Autodesk Inventor part; units mm, degrees
ref_plane "YZ Plane" through (0, 0, 0) normal (1, 0, 0) x (0, 1, 0)
ref_plane "XZ Plane" through (0, 0, 0) normal (0, 1, 0) x (-1, 0, 0)
ref_plane "XY Plane" through (0, 0, 0) normal (0, 0, 1) x (1, 0, 0)
sketch "Skizze1" plane through (0, 0, 0) normal (0, 0, 1) x (1, 0, 0)
  line L0 (27.5, 0) -> (-27.5, 0)
  line L1 (-27.5, 0) -> (-27.5, 210)
  line L2 (-27.5, 210) -> (27.5, 210)
  line L3 (27.5, 210) -> (27.5, 0)
  line L4 (0, 252) -> (0, -42)
  line L5 (-38.5, 0) -> (38.5, 0)
  point P0 (0, 0)
  point P1 (0, 0)
  dimension "d0" = 210
  dimension "d1" = 55
extrude "Extrusion1" add sketch "Skizze1" along normal blind 10
sketch "Skizze2" plane through (0, 0, 10) normal (0, 0, 1) x (1, 0, 0)
  line L0 (27.5, 210) -> (27.5, 0)
  circle A0 centre (3.5, 195.1) radius 4.3
  circle A1 centre (-6.5, 192.1) radius 1.2295
  circle A2 centre (-6.5, 198.1) radius 1.2295
  line L1 (21.5, 200.1) -> (-17.5, 200.1)
  line L2 (-17.5, 190.1) -> (-17.5, 200.1)
  line L3 (21.5, 190.1) -> (-17.5, 190.1)
  line L4 (21.5, 190.1) -> (21.5, 200.1)
  line L5 (19.1583, 143.6) -> (26.6417, 143.6)
  arc A3 (19.1583, 156.6) -> (19.1583, 143.6) centre (22.9, 150.1) ccw
  line L6 (26.6417, 156.6) -> (19.1583, 156.6)
  arc A4 (26.6417, 143.6) -> (26.6417, 156.6) centre (22.9, 150.1) ccw
  circle A5 centre (3.5, 105.1) radius 4.3
  circle A6 centre (-6.5, 102.1) radius 1.2295
  circle A7 centre (-6.5, 108.1) radius 1.2295
  line L7 (21.5, 110.1) -> (-17.5, 110.1)
  line L8 (-17.5, 100.1) -> (-17.5, 110.1)
  line L9 (21.5, 100.1) -> (-17.5, 100.1)
  line L10 (21.5, 100.1) -> (21.5, 110.1)
  line L11 (27.5, 200.4) -> (-15.4311, 200.4)
  line L12 (-15.4311, 189.8) -> (27.5, 189.8)
  line L13 (27.5, 189.8) -> (27.5, 200.4)
  arc A8 (-17.5, 191.8689) -> (-15.4311, 189.8) centre (-16.7, 190.6) ccw
  arc A9 (-15.4311, 200.4) -> (-17.5, 198.3311) centre (-16.7, 199.6) ccw
  line L14 (22.9, 150.1) -> (-7.7295, 150.1) construction
  line L15 (-17.5, 190.1) -> (-17.5, 189.8)
  line L16 (-17.5, 200.4) -> (-17.5, 200.1)
  line L17 (-17.5, 198.3311) -> (-17.5, 191.8689)
  circle A10 centre (3.5, 105.1) radius 4.3
  circle A11 centre (-6.5, 108.1) radius 1.2295
  circle A12 centre (-6.5, 102.1) radius 1.2295
  line L18 (21.5, 100.1) -> (-17.5, 100.1)
  line L19 (-17.5, 110.1) -> (-17.5, 100.1)
  line L20 (21.5, 110.1) -> (-17.5, 110.1)
  line L21 (21.5, 110.1) -> (21.5, 100.1)
  line L22 (27.5, 99.8) -> (-15.4311, 99.8)
  line L23 (-15.4311, 110.4) -> (27.5, 110.4)
  line L24 (27.5, 110.4) -> (27.5, 99.8)
  arc A13 (-15.4311, 110.4) -> (-17.5, 108.3311) centre (-16.7, 109.6) ccw
  arc A14 (-17.5, 101.8689) -> (-15.4311, 99.8) centre (-16.7, 100.6) ccw
  line L25 (-17.5, 110.1) -> (-17.5, 110.4)
  line L26 (-17.5, 99.8) -> (-17.5, 100.1)
  line L27 (-17.5, 101.8689) -> (-17.5, 108.3311)
  line L28 (27.5, 156.9) -> (18.4, 156.9)
  line L29 (15.4, 153.9) -> (15.4, 146.3)
  line L30 (18.4, 143.3) -> (27.5, 143.3)
  line L31 (27.5, 143.3) -> (27.5, 156.9)
  arc A15 (18.4, 156.9) -> (15.4, 153.9) centre (18.4, 153.9) ccw
  arc A16 (15.4, 146.3) -> (18.4, 143.3) centre (18.4, 146.3) ccw
  point P0 (0, 0)
  dimension "d4" = 0.3
  dimension "d5" = 0.3
  dimension "d6" = 3
  dimension "d7" = 3
  dimension "d8" = 0.8
  dimension "d9" = 0.8
  dimension "d10" = 0.8
  dimension "d11" = 0.8
  dimension "d13" = 10.6
  dimension "d15" = 0.3
  dimension "d16" = 0.3
  dimension "d17" = 12.1
  dimension "d18" = 3
extrude "Extrusion2" cut sketch "Skizze2" against normal through all contours L0 L22 A14 L8 L9 L10 L7 A13 L23 | L0 A4 L6 A3 L29 A15 L28 | L0 L12 A8 L2 L3 L4 L1 A9 L11 | L2 L1 L4 L3 | A4 L0 | L0 A4 L5 A3 L6 | L0 L30 A16 L29 A3 L5 A4 | L8 L7 L10 L9 | A0 | A1 | A2 | A5 | A6 | A7
sketch "Skizze3" plane through (-27.5, 0, 0) normal (0, -1, 0) x (1, 0, 0)
  line L0 (55, 10) -> (0, 10)
  line L1 (0, 0) -> (0, 10)
  point P0 (27.5, 0)
  point P1 (5, 5)
  point P2 (35, 5)
  dimension "d21" = 30
  dimension "d22" = 5
  dimension "d23" = 5
  dimension "d24" = 5
hole "Bohrung1" at (-22.5, 0, 5) at (7.5, 0, 5) direction (0, 1, 0) diameter 4.134 depth 15 tip angle 118
equation "\"d4\" = d5"
equation "\"d7\" = d6"
equation "\"d9\" = d8"
equation "\"d10\" = d8"
equation "\"d11\" = d10"
equation "\"d16\" = d15"
properties part number "Rückhalter" material "Stainless Steel"
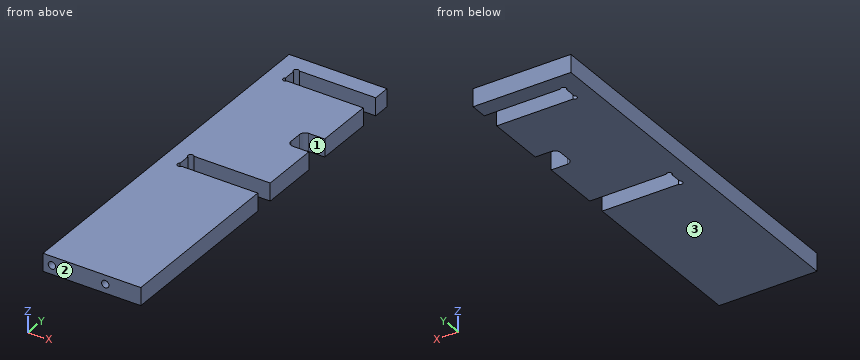
Input: part model. Units: mm. Frame: model coordinates. Face numbers are marked on the shaded views. Round coordinates to 2 decimals unless told otherwise and drop trailing zeros. Loops run counter-clockwise (first coordinate to the right, second up) from the corner with the lowest first, then second, coordinate; pieces in that order, holes last. Notation, with made-up numbers: (70.25, 11.25) - (113.25, 11.25) arc R18 ccw to (113.25, 15.25) - close; hole circle Ø10 at (10, -37). An arc over 180 degrees is marked (long way). One line per item, written item: value. Start each with the question number.
(1) Draft query along Y for the marked faces 1, 2 and 3. Return one class per face: +Y half, -Y half, draft (parallel to the pull), parting line (faces both ways), or undercut.
(2) Ray query, line 1 (Y direction, x = 20, z = 1.5); line 2 (Y direction, x = -6, z = 9); line 3 (Y direction, x = -16.7, z = 3.75). Return the intervals inside material, ascending. Write a range as [from, to].
(3) Section A-A, the plane x = 1. Return loops of the section in (y, z), plus the area to 3 significant figures.
(4) Contact query for flat-ended pins moving along their axis: P1, Ø10, axis at x = 16.5, y = 150, coming from the +Z side; P2, Ø5, axis at y = 104.5, z = 6.5, coming from the +X side; P3, Ø3.5, axis at x = -22.5, z = 5, coming from the -Y side; P4, Ø6, axis at y = 150, z = 4.5, coming from the +X side. Output: stop coordinate, or through.
Results below:
1. face 1: undercut
1. face 2: -Y half
1. face 3: draft
2. line 1: [0, 99.8], [110.4, 143.3], [156.9, 189.8], [200.4, 210]
2. line 2: [0, 99.8], [110.4, 189.8], [200.4, 210]
2. line 3: [0, 99.1], [111.1, 189.1], [201.1, 210]
3. outline: (0, 0) - (99.8, 0) - (99.8, 10) - (0, 10) - close; (110.4, 0) - (189.8, 0) - (189.8, 10) - (110.4, 10) - close; (200.4, 0) - (210, 0) - (210, 10) - (200.4, 10) - close
3. area: 1,890 mm^2
4. P1: z = 10
4. P2: x = -17.5
4. P3: y = 15.19
4. P4: x = 15.4
